Check sheet for the modelled part. Datum: model origin and axes. Units: mm. Face numbers are marked on the shaded views. Give positions to 0.01 mm unless a question says otherwise; leave off trailing zeros. Order: outer loops, then holes, each group sorted by start corner. A loop starts at its lowest first (then second) coordinate and runs counter-clockwise, first axis right, second up.
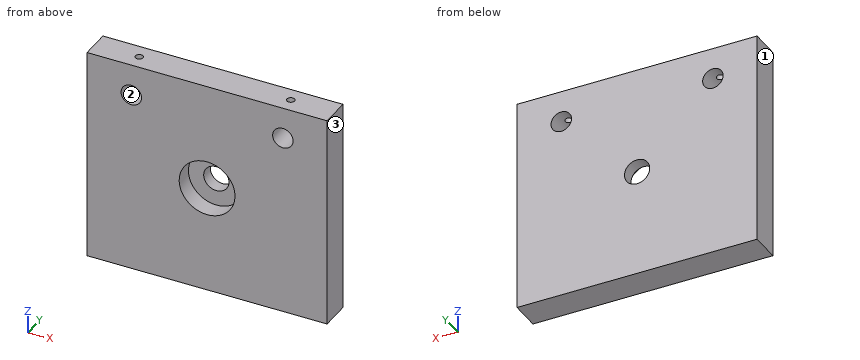
```python
from build123d import *

# Parameters (mm, degrees)
SKETCH1_W           = 95
SKETCH1_H           = 12
BOSS_EXTRUDE1_DEPTH = 85
SKETCH2_R           = 4.05
SKETCH2_R_2         = 5
CUT_EXTRUDE1_DEPTH  = 13
SKETCH3_R           = 11.05
CUT_EXTRUDE2_DEPTH  = 7
CUT_EXTRUDE3_REACH  = 87
SKETCH4_R           = 1.5


with BuildPart() as part:
    # Sketch1 → Boss-Extrude1 (new body)
    with BuildSketch(Plane.XY):
        Rectangle(SKETCH1_W, SKETCH1_H)
    extrude(amount=BOSS_EXTRUDE1_DEPTH)

    # Sketch2 → Cut-Extrude1 (cut, through all)
    with BuildSketch(Plane.XZ.offset(6)):
        with Locations(Location((-30, 72.5, 0), (0, 0, 270))):  # turned: the seam where the file's is
            Circle(SKETCH2_R)
        with Locations(Location((30, 72.5, 0), (0, 0, 270))):  # turned: the seam where the file's is
            Circle(SKETCH2_R)
        with Locations(Location((0, 42.5, 0), (0, 0, 270))):  # turned: the seam where the file's is
            Circle(SKETCH2_R_2)
    extrude(amount=-CUT_EXTRUDE1_DEPTH, mode=Mode.SUBTRACT)

    # Sketch3 → Cut-Extrude2 (cut)
    with BuildSketch(Plane.XZ.offset(6)):
        with Locations(Location((0, 42.5, 0), (0, 0, 270))):  # turned: the seam where the file's is
            Circle(SKETCH3_R)
    extrude(amount=-CUT_EXTRUDE2_DEPTH, mode=Mode.SUBTRACT)

    # Sketch4 → Cut-Extrude3 (cut, up to next)
    with BuildSketch(Plane.XY.offset(85), mode=Mode.PRIVATE) as cut_extrude3_sk1:
        with Locations((30, 0)):
            Circle(SKETCH4_R)
    cut_extrude3_tool1 = extrude(cut_extrude3_sk1.sketch, amount=-CUT_EXTRUDE3_REACH, mode=Mode.PRIVATE) & part.part
    add(cut_extrude3_tool1.solids().sort_by_distance((30, 0, 85))[0], mode=Mode.SUBTRACT)
    # Sketch4 → Cut-Extrude3 (cut, up to next)
    with BuildSketch(Plane.XY.offset(85), mode=Mode.PRIVATE) as cut_extrude3_sk2:
        with Locations((-30, 0)):
            Circle(SKETCH4_R)
    cut_extrude3_tool2 = extrude(cut_extrude3_sk2.sketch, amount=-CUT_EXTRUDE3_REACH, mode=Mode.PRIVATE) & part.part
    add(cut_extrude3_tool2.solids().sort_by_distance((-30, 0, 85))[0], mode=Mode.SUBTRACT)


solid = part.part
```
(1) Cross-section at D-D on z = 42.5. Enter the section's corners in (x, y).
Response values:
outline: (-47.5, -6) - (-11.05, -6) - (-11.05, 1) - (-5, 1) - (-5, 6) - (-47.5, 6) - close; (5, 1) - (11.05, 1) - (11.05, -6) - (47.5, -6) - (47.5, 6) - (5, 6) - close
(2) Cross-section at B-B on x = -30. Enter the section's corners in (y, z).
Response values:
outline: (-6, 0) - (6, 0) - (6, 68.45) - (-6, 68.45) - close; (-6, 76.55) - (-1.5, 76.55) - (-1.5, 85) - (-6, 85) - close; (1.5, 76.55) - (6, 76.55) - (6, 85) - (1.5, 85) - close
(3) Release check for a two-part mould opening along X. For the marked faces 1, 2 and 3 record: released by +X, released by -X, zero draft, split by the parting line, or undercut.
Response values:
face 1: released by -X
face 2: undercut
face 3: released by +X
(4) Cross-section at A-A on z = 72.5. Enter the section's corners in (x, y), then the cut area to 3 significant figures.
Response values:
outline: (-47.5, -6) - (-34.05, -6) - (-34.05, 6) - (-47.5, 6) - close; (-25.95, -6) - (25.95, -6) - (25.95, 6) - (-25.95, 6) - close; (34.05, -6) - (47.5, -6) - (47.5, 6) - (34.05, 6) - close
area: 946 mm2
(5) Material ranges on L1, parallel to X at y = 0, z = 82.25; L2, parallel to X at y = 3, z = 72.5; L3, parallel to X at y = -2, z = 42.5, recorded low to high.
Response values:
L1: x = -47.5 to -31.5, -28.5 to 28.5, 31.5 to 47.5
L2: x = -47.5 to -34.05, -25.95 to 25.95, 34.05 to 47.5
L3: x = -47.5 to -11.05, 11.05 to 47.5
(6) Gauge pin test, flat ends, axial feed: pin 1 Ø2.5 at (x, y) = (30, 0) entering from +Z; pin 2 Ø7.5 at (x, z) = (-30, 72.5) entering from +Y; pin 3 Ø11 at (x, z) = (3, 40.5) entering from -Y. Record the tip position at first contact, or that the pin passes through.
Response values:
pin 1: stops at z = 68.65
pin 2: passes through
pin 3: stops at y = 1
(7) Cross-section at C-C on y = -3. Enter the section's corners in (x, z).
Response values:
outline: (-47.5, 0) - (47.5, 0) - (47.5, 85) - (-47.5, 85) - close; hole circle Ø8.1 at (-30, 72.5); hole circle Ø22.1 at (0, 42.5); hole circle Ø8.1 at (30, 72.5)
